```python
from build123d import *

# Parameters (mm, degrees)
F0_R     = 7.5
F0_R_2   = 1
F1_DEPTH = 7
F2_DEPTH = 5
F3_R     = 2.5


with BuildPart() as f1:
    # F0 (on Top) → F1 (new body)
    with BuildSketch(Plane.XY):
        Circle(F0_R)
        Circle(F0_R_2, mode=Mode.SUBTRACT)
    extrude(amount=F1_DEPTH)

    # F0 (on Top) → F2 (join)
    with BuildSketch(Plane.XY):
        Circle(F0_R)
        Circle(F0_R_2, mode=Mode.SUBTRACT)
    extrude(amount=F2_DEPTH)

    # F3
    f3_edges = [f1.edges().sort_by_distance(p)[0] for p in [
        (-7.5, 0, 7),
        (-7.5, 0, 0),
    ]]
    fillet(f3_edges, radius=F3_R)


solid = f1.part
```
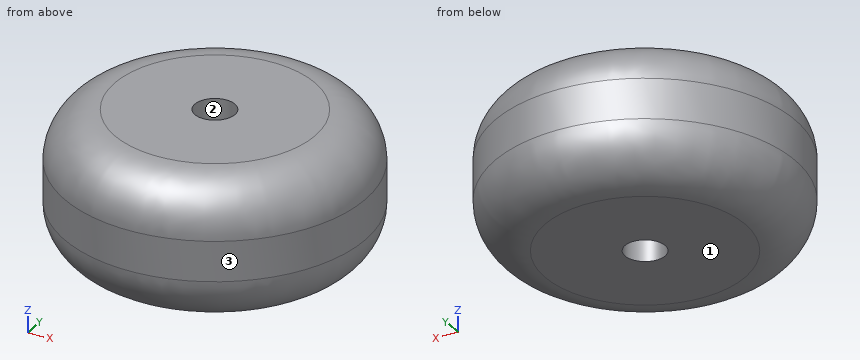
Can you work these out from the model? Positions are in its coordinate system, mm. Face numbers are marked on the shaded views. Coordinates: 2 decimals unless noted, no trailing zeros. Loops run counter-clockwise (first coordinate to the right, second up) from the corner with the lowest first, then second, coordinate; pieces in that order, holes last. Notation, with made-up numbers: (70, 71) -> (105, 71) arc R9 cw to (105, 85) -> close; hole circle Ø4 at (77.25, -21.5). An arc over 180 degrees is marked (long way). Put each result on its own line as item: value. Start each with the question number.
Q1. I'm going to push flat-ended pins straight in: P1, Ø1, axis at x = -3, z = 3.5, coming from the -Y side; P2, Ø2, axis at x = -1, z = 5.5, coming from the +Y side; P3, Ø2, axis at x = -0.5, z = 4, coming from the -Y side; P4, Ø2, axis at x = 0.5, z = 1, coming from the +Y side. Where does each tip first touch, or does it pass through?
Q2. I want a section at A-A (x = 0). Write out the boundary of the cut face in (y, z), plus the area to 3 significant figures.
Q3. I want a section at C-C (z = 3.25). Write out the boundary of the cut face in (x, y).
Q4. Thinking about a two-plate mould opening in X: for the marked faces 1, 2 and 3, which applies, pulls with the +X half, pulls with the -X half, needs draft (parallel to the pull), parting line crosses it, or undercut?
Q5. If I drill on line 1 (Y direction, x = 0, z = 3); line 2 (Y direction, x = 0, z = 5.25); line 3 (X direction, y = -2.25, z = 5.25), over which ranges is the centre line in solid material (lowest first)? Write a range as [from, to].
Q6. I want a section at D-D (z = 5.25). Write out the boundary of the cut face in (x, y), plus the area to 3 significant figures.
Taken from the geometry:
1. P1: stops at y = -7.07
1. P2: stops at y = 7.48
1. P3: stops at y = -7.5
1. P4: stops at y = 7.44
2. outline: (-7.5, 2.5) arc R2.5 ccw to (-5, 0) -> (-1, 0) -> (-1, 7) -> (-5, 7) arc R2.5 ccw to (-7.5, 4.5) -> close; (1, 0) -> (5, 0) arc R2.5 ccw to (7.5, 2.5) -> (7.5, 4.5) arc R2.5 ccw to (5, 7) -> (1, 7) -> close
2. area: 85.6 mm2
3. outline: circle Ø15 at (0, 0); hole circle Ø2 at (0, 0)
4. face 1: needs draft
4. face 2: undercut
4. face 3: parting line crosses it
5. line 1: y = [-7.5, -1], [1, 7.5]
5. line 2: y = [-7.38, -1], [1, 7.38]
5. line 3: x = [-7.03, 7.03]
6. outline: circle Ø14.77 at (0, 0); hole circle Ø2 at (0, 0)
6. area: 168 mm2
